For this review, use the dimensioned drawing (mm, ordinates from the lowest corner) and the shaded views. A direction names the side the tool comes from. Give positions to 0.01 mm unless a question says otherwise; leave off trailing zeros. Loops run counter-clockwise (first coordinate to the right, second up) from the corner with the lowest first, then second, coordinate; pieces in that order, holes last. Notation, with made-up numbers: M -35,-22.75 L 10,-22.75 A26 cw 10,3.25 Z; hole C -26,-32.75 d7. An arc over 180 degrees is marked long. Return JSON: item names as keys, results as strings.
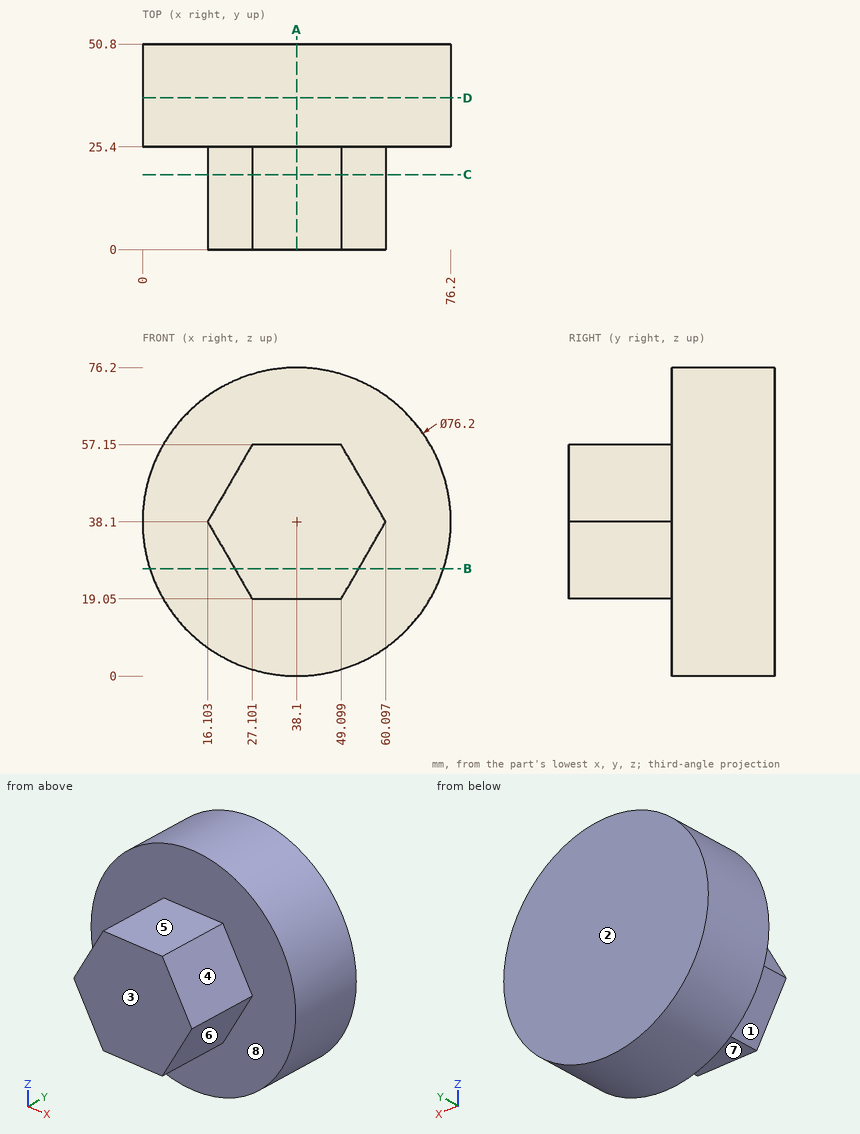
1) The part is to be moulded in two halves that separate along Y. For the marked faces 1, 2 and 3, say which applies: released by +Y, released by -Y, zero draft, split by the parting line, or undercut.
From the geometry:
{"face 1": "zero draft", "face 2": "released by +Y", "face 3": "released by -Y"}
2) Tool access review of the marked faces 4, 5, 6, 7 and 8: name each direction out of +Z, -Z, +X, -X, +Y, -Y from which nothing blocks a thin tool from reaching the whole face with its end or side.
From the geometry:
{"face 4": "+Z, +X, -Y", "face 5": "+Z, +X, -X, -Y", "face 6": "-Z, +X, -Y", "face 7": "-Z, +X, -X, -Y", "face 8": "-Y"}
3) Consider section B-B on z = 26.5. Write out the cut boundary in (x, y).
From the geometry:
{"outline": "M 1.81,25.4 L 22.8,25.4 L 22.8,0 L 53.4,0 L 53.4,25.4 L 74.39,25.4 L 74.39,50.8 L 1.81,50.8 Z"}
4) Consider section D-D on y = 37.5. Write out the cut boundary in (x, z).
From the geometry:
{"outline": "C 38.1,38.1 d76.2"}
5) Consider section A-A on x = 38.1. Write out the cut boundary in (y, z), then the cut area to 3 significant figures.
From the geometry:
{"outline": "M 0,19.05 L 25.4,19.05 L 25.4,0 L 50.8,0 L 50.8,76.2 L 25.4,76.2 L 25.4,57.15 L 0,57.15 Z", "area": "2,900 mm²"}
6) Wall thickness on L1, parallel to Z at x = 41, y = 10; L2, parallel to Y at x = 14, z = 17; L3, parallel to Z at x = 14.5, y = 38.5: over which ranges is each line inside the solid? List them lowest first. Write a range as from..to.
From the geometry:
{"L1": "19.05..57.15", "L2": "25.4..50.8", "L3": "8.19..68.01"}
7) Insertion check: pin 1 (4 mm diameter, centred on x = 64, z = 24.5, fed in from -Y); pin 2 (4 mm diameter, centred on y = 7, z = 33, fed in from -X); pin 3 (6 mm diameter, centred on x = 49, y = 23.5, fed in from +Z); pin 4 (23 mm diameter, centred on x = 34, z = 39.5, fed in from -Y). Each pin has a flat end and moves straight along its axis. Give the tip position at first contact, or say it passes through.
From the geometry:
{"pin 1": "y = 25.4", "pin 2": "x = 17.89", "pin 3": "z = 75.22", "pin 4": "y = 0"}
8) Consider section C-C on y = 18.5. Write out the cut boundary in (x, z), then the cut area to 3 significant figures.
From the geometry:
{"outline": "M 16.1,38.1 L 27.1,19.05 L 49.1,19.05 L 60.1,38.1 L 49.1,57.15 L 27.1,57.15 Z", "area": "1,260 mm²"}
